CAD build for the part. Positions are in the model's coordinates, mm. A direction names the side the tool comes from. Give positions to 0.01 mm unless a question says otherwise; leave off trailing zeros. Order: outer loops, then holes, each group sorted by start corner. A loop starts at its lowest first (then second) coordinate and runs counter-clockwise, first axis right, second up.
```python
from build123d import *

# Parameters (mm, degrees)
PATTERN_CIRCULAR_1_COUNT = 4


with BuildPart() as part:
    # 草图2 → 旋转1 (revolve)
    with BuildSketch(Plane(origin=(0, 0, 0), x_dir=(0, 0, -1), z_dir=(1, 0, 0))):
        Polygon((-2, 1.5), (-2, 10), (0, 10), (0, 5), (3.5, 5), (3.5, 3), (0, 3), (0, 1.5), align=None)
    revolve(axis=Axis((0, 0, 0), (0, 0, 1)))

    # 草图4 → M3 螺纹孔1 (revolve, cut)
    with BuildSketch(Plane(origin=(0, 7, 2), x_dir=(0, -1, 0), z_dir=(1, 0, 0))):
        Polygon((0, 0), (0, 8.251075774), (1.25, 7.5), (1.25, 0), align=None)
    hole_wizard_m3_1 = revolve(axis=Axis((0, 7, 8.35), (0, 0, -1)), mode=Mode.SUBTRACT)

    # 阵列(圆周)1: M3 螺纹孔1 ×4 about axis
    pattern_circular_1_axis = Axis((0, 0, 0), (0, 0, 1))
    for i in range(1, PATTERN_CIRCULAR_1_COUNT):
        add(hole_wizard_m3_1.rotate(pattern_circular_1_axis, i * 360 / PATTERN_CIRCULAR_1_COUNT), mode=Mode.SUBTRACT)


solid = part.part
```
Item 1: Two-plate mould, pull along X, no slides. Class faces 3 (the face through (1.3, 1.3, 0)), 4 (the face through (-5, 2, 0)), 5 (the face through (9.76, -2.17, 0.99)): released by +X, released by -X, zero draft, split by the parting line, or undercut.
Item 2: Slice it at C-C (z = 0.6). Give the cut face in (x, y).
Item 3: Tool access for faces 1 (the face through (-0.07, -1.5, 1.01)), 2 (the face through (4.88, -1.08, -1.77)): list every direction of +Z, -Z, +X, -X, +Y, -Y with a clear straight run to the whole face (end or side of a thin tool).
Item 4: Drop flat-ended pins along their axis: pin 1 Ø3 at (x, z) = (-2.5, -1) entering from -Y; pin 2 Ø3 at (x, y) = (7, 0) entering from -Z. Give the stop position or say it passes through.
Item 5: Slice it at A-A (x = 0). Give the cut face in (y, z).
Item 6: Wall check: L1, parallel to Y at x = 0, z = 1.05; L2, parallel to Y at x = 0, z = -1.8; L3, parallel to Z at x = 1.75, y = 1. Give the ranges that are in metal, low to high.
Item 7: Slice it at D-D (y = -7). Give the cut face in (x, z).
A:
1. face 3: undercut
1. face 4: zero draft
1. face 5: split by the parting line
2. outline: circle Ø20 at (0, 0); hole circle Ø2.5 at (-7, 0); hole circle Ø3 at (0, 0); hole circle Ø2.5 at (0, -7); hole circle Ø2.5 at (0, 7); hole circle Ø2.5 at (7, 0)
3. face 1: +Z, -Z
3. face 2: -Z
4. pin 1: stops at y = -9.9
4. pin 2: stops at z = 0
5. outline: (-10, 0) - (-8.25, 0) - (-8.25, 2) - (-10, 2) - close; (-5.75, 0) - (-5, 0) - (-5, -3.5) - (-3, -3.5) - (-3, 0) - (-1.5, 0) - (-1.5, 2) - (-5.75, 2) - close; (1.5, 0) - (3, 0) - (3, -3.5) - (5, -3.5) - (5, 0) - (5.75, 0) - (5.75, 2) - (1.5, 2) - close; (8.25, 0) - (10, 0) - (10, 2) - (8.25, 2) - close
6. L1: y = -10 to -8.25, -5.75 to -1.5, 1.5 to 5.75, 8.25 to 10
6. L2: y = -5 to -3, 3 to 5
6. L3: z = 0 to 2
7. outline: (-7.14, 0) - (-1.25, 0) - (-1.25, 2) - (-7.14, 2) - close; (1.25, 0) - (7.14, 0) - (7.14, 2) - (1.25, 2) - close
